from build123d import *

# Parameters (mm, degrees)
F1_DEPTH = 63.5
F2_R     = 6.4197594032
F3_DEPTH = 23.4593788755
F4_W     = 124.8833438046
F4_H     = 12.7
F5_DEPTH = 6.35
F6_R     = 2.54


with BuildPart() as f1:
    # F0 (on Front) → F1 (new body)
    with BuildSketch(Plane.XZ):
        Polygon((58.006938024, -82.3166997439), (39.3296977039, -93.179662284), (-7.1721252495, -13.2267286881), (-10.8084349941, -20.9649698821), (-50.382357985, -105.180172272), (-37.2205925623, -105.180172272), (-7.1087183348, -41.1006625658), (30.1608836833, -105.180172272), (46.3093739423, -105.180172272), (65.3555968279, -94.9516200987), align=None)
    extrude(amount=F1_DEPTH)

    # F2 (on face) → F3 (cut, through all)
    with BuildSketch(Plane(origin=(50.4372636726, 0, -86.7193356531), x_dir=(0.8644246839, 0, 0.5027623353), z_dir=(-0.5027623353, 0, 0.8644246839))):
        with Locations((-3.9596631056, -31.75)):
            Circle(F2_R)
    extrude(amount=-F3_DEPTH, mode=Mode.SUBTRACT)

    # F4 (on face) → F5 (cut)
    with BuildSketch(Plane(origin=(0, 0, -105.180172272), x_dir=(1, 0, 0), z_dir=(0, 0, -1))):
        with Locations((11.0299456865, 31.75)):
            Rectangle(F4_W, F4_H)
    extrude(amount=-F5_DEPTH, mode=Mode.SUBTRACT)

    # F6
    f6_edges = [f1.edges().sort_by_distance(p)[0] for p in [
        (-7.172125, -31.75, -13.226729),
        (16.078786, -63.5, -53.203195),
        (16.078786, 0, -53.203195),
        (-28.777242, -63.5, -59.20345),
        (-28.777242, 0, -59.20345),
    ]]
    fillet(f6_edges, radius=F6_R)


solid = f1.part
The model under review builds one solid part; all positions refer to its coordinate system, in mm. A direction names the side the tool comes from. Round coordinates to 2 decimals unless told otherwise and drop trailing zeros. Loops run counter-clockwise (first coordinate to the right, second up) from the corner with the lowest first, then second, coordinate; pieces in that order, holes last. Notation, with made-up numbers: (-32.75, -2) -> (14.25, -2) arc R16 cw to (14.25, 23) -> close; hole circle Ø2 at (37, 31.25). An arc over 180 degrees is marked (long way). Write item = value, one per line. Start each with the question number.
Item 1: To check wall thickness, follow L1, parallel to X at y = -29, z = -97; L2, parallel to X at y = -40, z = -99.5; L3, parallel to X at y = -58, z = -95.5. State the ranges of each line that lie inside material, in increasing order.
Item 2: Insertion check: pin 1 (0.5 mm diameter, centred on x = 56.5, y = -26, fed in from -Z); pin 2 (6 mm diameter, centred on y = -33.5, z = -53.5, fed in from +X); pin 3 (1 mm diameter, centred on y = -40.5, z = -31, fed in from +X). Each pin has a flat end and moves straight along its axis. Give the tip position at first contact, or say it passes through.
Item 3: For faces 4 (the flat face through (-41, -32, -98.83)), 5 (the flat face through (38, -51, -105.18)), list the 3-axis set-ups (+Z, -Z, +X, -X, +Y, -Y) from which the entire face can be reached by the end or side of a thin tool; tool diameter is ignored.
Item 4: Take a section at B-B on z = -91.5. Count the separate pieces of the cut face and the enclosed holes in it, plus the area to 3 significant figures.
Item 5: Mouldability with a two-part tool opening along Y and no side actions: class faces 1 (the flat face through (11.265, -31.306, -72.692)), 2 (the flat face through (9, 0, -68)), 3 (the flat face through (40, -38.1, -102)) as released by +Y, released by -Y, zero draft, split by the parting line, or undercut.
Item 6: Take a section at A-A on y = -56. Give the boundary of the cut face in (x, z), plus the area to 3 significant figures.
Result:
q1.L1 = -46.54 to -33.38, 25.4 to 45.13, 58.55 to 61.54
q1.L2 = -47.71 to -34.55, 26.86 to 56.89
q1.L3 = -45.83 to -32.67, 24.53 to 64.33
q2.pin_1 = -98.83
q2.pin_2 = 18
q2.pin_3 = 3.46
q3.face_4 = -Z, +X, -X
q3.face_5 = -Z, +X, -X, +Y, -Y
q4.separate_pieces = 3
q4.enclosed_holes = 0
q4.area = 3,050 mm²
q5.face_1 = zero draft
q5.face_2 = released by +Y
q5.face_3 = undercut
q6.outline = (-50.38, -105.18) -> (-37.22, -105.18) -> (-7.11, -41.1) -> (30.16, -105.18) -> (46.31, -105.18) -> (65.36, -94.95) -> (58.01, -82.32) -> (39.33, -93.18) -> (-4.74, -17.41) arc R2.54 ccw to (-9.23, -17.61) -> close
q6.area = 2,590 mm²
